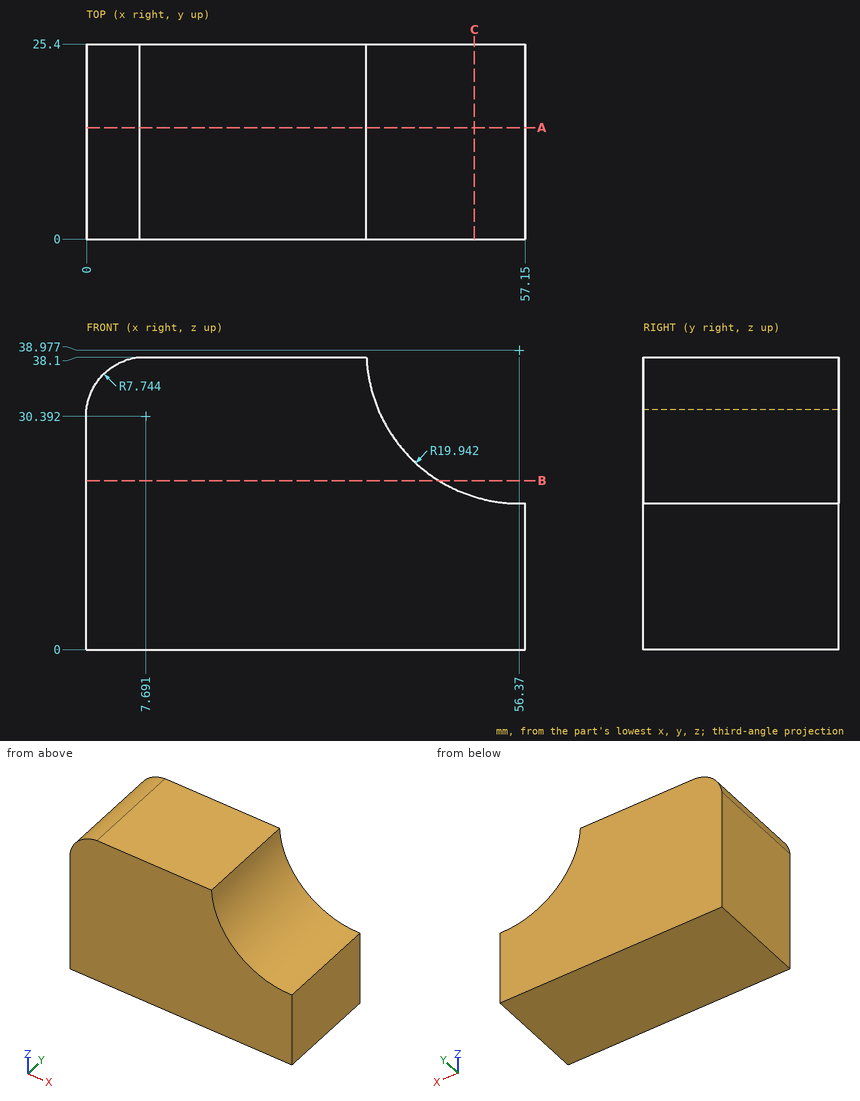
Here's the drawing with two shaded views (mm, measured from the low corner). I have some questions. Give positions to 0.01 mm unless a question says otherwise; leave off trailing zeros. Loops run counter-clockwise (first coordinate to the right, second up) from the corner with the lowest first, then second, coordinate; pieces in that order, holes last. Notation, with made-up numbers: (53, 4.25) -> (60, 4.25) arc R29 ccw to (60, 42.25) -> close; hole circle Ø7 at (34, 54). An arc over 180 degrees is marked (long way). Answer as a JSON object with one key per item and string values. Group by question number.
Item 1: Imagine slicing it at A-A on y = 14.5. Write out the boundary of the cut face in (x, z).
Item 2: I need wall thicknesses on L1, parallel to Z at x = 46, y = 3.25; L2, parallel to Z at x = 52, y = 17; L3, parallel to X at y = 24, z = 36.5. Which ranges of each line are inside material? Lowest first, please.
Item 3: Imagine slicing it at B-B on z = 22. Write out the boundary of the cut face in (x, y).
Item 4: Will these pins go through, and if not, where does the flat tip stop? pin 1 (6 mm diameter, centred on y = 20.5, z = 33, fed in from +X); pin 2 (5 mm diameter, centred on x = 20.5, y = 13.5, fed in from -Z).
Item 5: Imagine slicing it at C-C on x = 50.5. Write out the boundary of the cut face in (y, z).
Answer list:
{
 "1": {"outline": "(0, 0) -> (57.15, 0) -> (57.15, 19.05) arc R19.94 cw to (36.45, 38.1) -> (6.94, 38.1) arc R7.74 ccw to (0, 31.3) -> close"},
 "2": {"L1": "z = 0 to 21.94", "L2": "z = 0 to 19.52", "L3": "x = 2.93 to 36.58"},
 "3": {"outline": "(0, 0) -> (45.91, 0) -> (45.91, 25.4) -> (0, 25.4) -> close"},
 "4": {"pin 1": "stops at x = 38.56", "pin 2": "stops at z = 0"},
 "5": {"outline": "(0, 0) -> (25.4, 0) -> (25.4, 19.92) -> (0, 19.92) -> close"}
}
